from build123d import *

# Parameters (mm, degrees)
SKETCH_1_R          = 2.1
SKETCH_1_R_2        = 2.65
SKETCH_1_R_3        = 2.6
EXTRUDE_1_DEPTH     = 3
FILLET_1_R          = 2
SKETCH_2_R          = 5.25
CUT_EXTRUDE_1_DEPTH = 1


with BuildPart() as part:
    # 草图1 → 凸台-拉伸1 (new body)
    with BuildSketch(Plane.XY):
        Polygon((14, 20), (14, 28), (37, 28), (37, -10), (-37, -10), (-37, 28), (-14, 28), (-14, 20), align=None)
        with Locations((17.5, 24)):
            Circle(SKETCH_1_R, mode=Mode.SUBTRACT)
        with Locations((25, 24)):
            Circle(SKETCH_1_R, mode=Mode.SUBTRACT)
        with Locations((32.5, 24)):
            Circle(SKETCH_1_R, mode=Mode.SUBTRACT)
        with Locations(Location((-32.5, 24, 0), (0, 0, 180))):
            Circle(SKETCH_1_R, mode=Mode.SUBTRACT)
        with Locations(Location((-17.5, 24, 0), (0, 0, 180))):
            Circle(SKETCH_1_R, mode=Mode.SUBTRACT)
        with Locations(Location((-25, 24, 0), (0, 0, 180))):
            Circle(SKETCH_1_R, mode=Mode.SUBTRACT)
        with Locations((30, 0)):
            Circle(SKETCH_1_R_2, mode=Mode.SUBTRACT)
        with Locations((-30, 0)):
            Circle(SKETCH_1_R_2, mode=Mode.SUBTRACT)
        with Locations((15, 5)):
            Circle(SKETCH_1_R_3, mode=Mode.SUBTRACT)
        with Locations((15, -5)):
            Circle(SKETCH_1_R_3, mode=Mode.SUBTRACT)
        with Locations(Location((-15, 5, 0), (0, 0, 180))):
            Circle(SKETCH_1_R_3, mode=Mode.SUBTRACT)
        with Locations(Location((-15, -5, 0), (0, 0, 180))):
            Circle(SKETCH_1_R_3, mode=Mode.SUBTRACT)
    extrude(amount=EXTRUDE_1_DEPTH)

    # 圆角1
    fillet_1_edges = [part.edges().sort_by_distance(p)[0] for p in [
        (14, 20, 1.5),
        (14, 28, 1.5),
        (37, 28, 1.5),
        (-37, 28, 1.5),
        (-14, 28, 1.5),
        (-14, 20, 1.5),
    ]]
    fillet(fillet_1_edges, radius=FILLET_1_R)

    # 草图2 → 切除-拉伸1 (cut)
    with BuildSketch(Plane.XY.offset(3)):
        with Locations((30, 0)):
            Circle(SKETCH_2_R)
        with Locations((-30, 0)):
            Circle(SKETCH_2_R)
    extrude(amount=-CUT_EXTRUDE_1_DEPTH, mode=Mode.SUBTRACT)


solid = part.part
Model file for the job. Use its own axes, mm. A direction names the side the tool comes from. Give positions to 0.01 mm unless a question says otherwise; leave off trailing zeros. Order: outer loops, then holes, each group sorted by start corner. A loop starts at its lowest first (then second) coordinate and runs counter-clockwise, first axis right, second up. Notation, with made-up numbers: (-2, 27.25) -> (55, 27.25) arc R20 ccw to (55, 49.25) -> close; hole circle Ø11 at (-6, 58.25). An arc over 180 degrees is marked (long way). Use CSV: the item, a comma, the result in double quotes.
1. Drop flat-ended pins along their axis: pin 1 (4 mm diameter, centred on x = -25, y = 24, fed in from +Z); pin 2 (1.5 mm diameter, centred on x = 7, z = 1.5, fed in from +Y); pin 3 (5 mm diameter, centred on x = -32.5, y = -1, fed in from +Z). Give the stop position or say it passes through.
Outcome:
pin 1,"through"
pin 2,"y = 20"
pin 3,"z = 2"
2. Band-saw the part on D-D, the plane x = 24. Give the cut face in (y, z), then the cut area to 3 significant figures.
Outcome:
outline,"(-10, 0) -> (22.15, 0) -> (22.15, 3) -> (-10, 3) -> close; (25.85, 0) -> (28, 0) -> (28, 3) -> (25.85, 3) -> close"
area,"103 mm²"
3. Drill centre lines: line 1 along X through (y, z) = (5.5, 1); line 2 along Y through (x, z) = (-15, 1.85); line 3 along Y through (x, z) = (-31, 2.35). Where is each one in solid material? Low to high. Write a range as from..to.
Outcome:
line 1,"-37..-17.55, -12.45..12.45, 17.55..37"
line 2,"-10..-7.6, -2.4..2.4, 7.6..27.73"
line 3,"-10..-5.15, 5.15..22.53, 25.47..28"
4. 3-axis set-ups, long thin cutter, end or side, ignore diameter. For faces 1 (the flat face through (32, -2, 2)), 2 (the cylindrical face through (17.48, -4.22, 1.48)), 3 (the cylindrical face through (-14.57, 27.4, 1.52)): which of +Z, -Z, +X, -X, +Y, -Y reach the whole face in a straight line?
Outcome:
face 1,"+Z"
face 2,"+Z, -Z"
face 3,"+Z, -Z, +Y"
5. Mould opens along X. For faces 4 (the flat face through (1, 9, 0)), 5 (the flat face through (37, 8, 1)), 6 (the cylindrical face through (-17.48, -5.78, 1.48)) say: +X half, -X half, draft (parallel to the pull), parting line (faces both ways), or undercut.
Outcome:
face 4,"draft"
face 5,"+X half"
face 6,"undercut"
6. Band-saw the part on C-C, the plane y = 0. Give the cut face in (x, z), then the cut area to 3 significant figures.
Outcome:
outline,"(-37, 0) -> (-32.65, 0) -> (-32.65, 2) -> (-35.25, 2) -> (-35.25, 3) -> (-37, 3) -> close; (-27.35, 0) -> (27.35, 0) -> (27.35, 2) -> (24.75, 2) -> (24.75, 3) -> (-24.75, 3) -> (-24.75, 2) -> (-27.35, 2) -> close; (32.65, 0) -> (37, 0) -> (37, 3) -> (35.25, 3) -> (35.25, 2) -> (32.65, 2) -> close"
area,"180 mm²"
7. Band-saw the part on A-A, the plane y = 24. Count the separate pieces of the cut face and the enclosed holes in it, then the cut area to 3 significant figures.
Outcome:
separate pieces,"8"
enclosed holes,"0"
area,"62.4 mm²"
